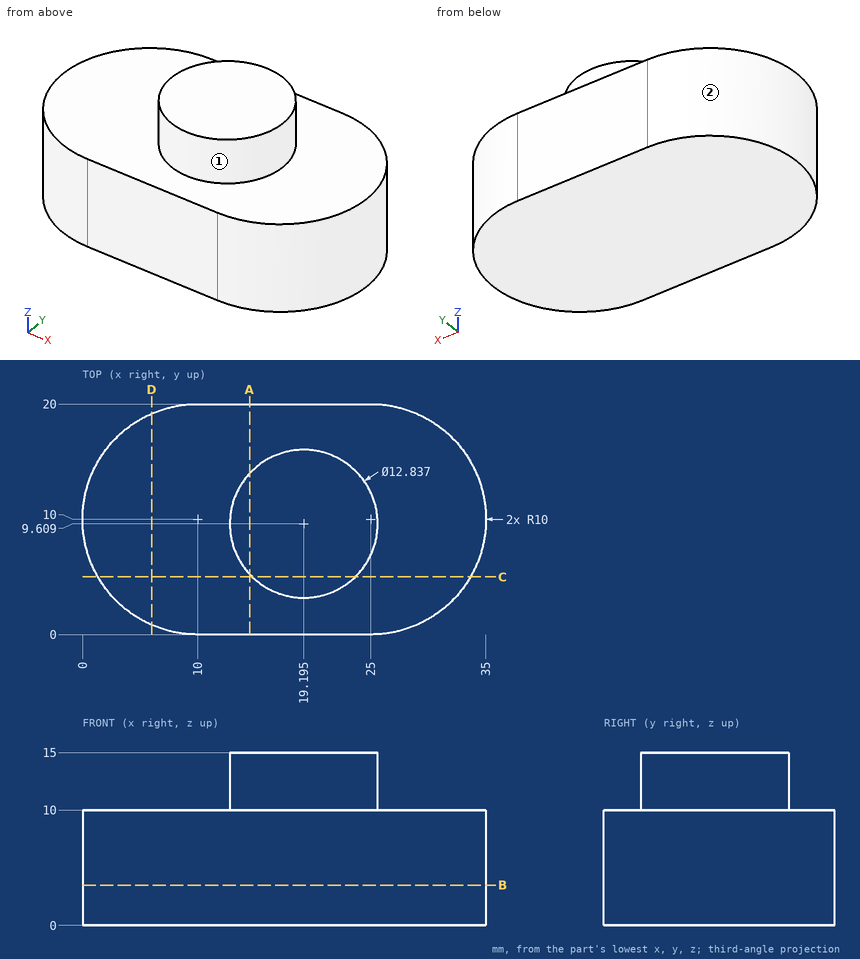
Answer from the drawing. Dimensions are ordinates in mm from the lowest x, y and z of the part. A direction names the side the tool comes from. Give positions to 0.01 mm unless a question says otherwise; leave off trailing zeros. Write each loop counter-clockwise with the first axis right and the second up, starting at its lowest first coordinate (ties: lowest second). Pieces come first, ordered by that corner, then holes. Notation, with made-up numbers: (60, 49.25) - (94, 49.25) arc R25 ccw to (94, 73.25) - close; hole circle Ø4 at (87.25, 27.25). An arc over 180 degrees is marked (long way). One line per item, written item: value. Start each with the question number.
1. Find section A-A (x = 14.5). Write down the section's boundary in (y, z) (1 decimal), then the cut area to 3 significant figures.
2. Consider probe 1 along Z at (x, y) = (12, 13.75); probe 2 along X at (y, z) = (8, 8.75); probe 3 along X at (y, z) = (1.5, 9.75). Determine where each line is inside the solid, lowest interval first.
3. Given pin 1 (3 mm diameter, centred on x = 25, z = 12, fed in from +Y); pin 2 (10 mm diameter, centred on x = 7, y = 14, fed in from +Z), each flat-ended and moving along its own axis, determine where each tip first touches the part or whether it passes through.
4. Find section C-C (y = 5). Write down the section's boundary in (x, z), then the cut area to 3 significant figures.
5. Find section B-B (z = 3.5). Write down the section's boundary in (x, y), then the cut area to 3 significant figures.
6. For the marked faces 1 and 2, determine the directions among +Z, -Z, +X, -X, +Y, -Y from which every point of the face is accessible in a straight line to the end or side of a thin tool.
7. Find section D-D (x = 6). Write down the section's boundary in (y, z) (1 decimal).
Geometry results:
1. outline: (0, 0) - (20, 0) - (20, 10) - (14, 10) - (14, 15) - (5.2, 15) - (5.2, 10) - (0, 10) - close
1. area: 244 mm2
2. probe 1: 0 to 10
2. probe 2: 0.2 to 34.8
2. probe 3: 4.73 to 30.27
3. pin 1: y = 14.37
3. pin 2: z = 10
4. outline: (1.34, 0) - (33.66, 0) - (33.66, 10) - (23.66, 10) - (23.66, 15) - (14.73, 15) - (14.73, 10) - (1.34, 10) - close
4. area: 368 mm2
5. outline: (10, 0) - (25, 0) arc R10 ccw to (25, 20) - (10, 20) arc R10 ccw to start
5. area: 614 mm2
6. face 1: +Z
6. face 2: +Z, -Z, -X
7. outline: (0.8, 0) - (19.2, 0) - (19.2, 10) - (0.8, 10) - close
